from build123d import *

# Parameters (mm, degrees)
F0_R     = 11.176
F1_DEPTH = 19.05
F0_R_2   = 6.35
F2_DEPTH = 12.7
F4_DEPTH = 31.75
F6_DEPTH = 16.002


with BuildPart() as f1:
    # F0 (on Front) → F1 (new body)
    with BuildSketch(Plane.XZ):
        with BuildLine():
            ThreePointArc((-25.4, -44.45), (-17.960512, -62.410512), (0, -69.85))
            ThreePointArc((0, -69.85), (17.960512, -62.410512), (25.4, -44.45))
            Line((25.4, -44.45), (25.4, 44.45))
            ThreePointArc((25.4, 44.45), (17.960512, 62.410512), (0, 69.85))
            ThreePointArc((0, 69.85), (-17.960512, 62.410512), (-25.4, 44.45))
            Line((-25.4, 44.45), (-25.4, -44.45))
        make_face()
        with Locations((0, -44.45)):
            Circle(F0_R, mode=Mode.SUBTRACT)
        with Locations((0, 44.45)):
            Circle(F0_R, mode=Mode.SUBTRACT)
    extrude(amount=F1_DEPTH)

    # F0 (on Front) → F2 (join)
    with BuildSketch(Plane.XZ):
        with Locations((0, -44.45)):
            Circle(F0_R)
        with Locations((0, -44.45)):
            Circle(F0_R_2, mode=Mode.SUBTRACT)
        with Locations((0, 44.45)):
            Circle(F0_R)
        with Locations((0, 44.45)):
            Circle(F0_R_2, mode=Mode.SUBTRACT)
    extrude(amount=F2_DEPTH)

    # F3 (on face) → F4 (join)
    with BuildSketch(Plane.XZ.offset(19.05)):
        with BuildLine():
            ThreePointArc((12.869681, 6.35), (13.975765, 3.260246), (14.351, 0))
            ThreePointArc((14.351, 0), (13.975765, -3.260246), (12.869681, -6.35))
            Line((12.869681, -6.35), (24.593444, -6.35))
            ThreePointArc((24.593444, -6.35), (24.631158, -6.2021), (24.667983, -6.053976))
            ThreePointArc((24.667983, -6.053976), (25.399541, 0.152632), (24.593444, 6.35))
            Line((24.593444, 6.35), (12.869681, 6.35))
        make_face()
        with BuildLine():
            ThreePointArc((6.35, 12.869681), (10.147689, 10.147689), (12.869681, 6.35))
            Line((12.869681, 6.35), (24.593444, 6.35))
            ThreePointArc((24.593444, 6.35), (17.960512, 17.960512), (6.35, 24.593444))
            Line((6.35, 24.593444), (6.35, 12.869681))
        make_face()
        with BuildLine():
            Line((24.593444, -6.35), (12.869681, -6.35))
            ThreePointArc((12.869681, -6.35), (10.147689, -10.147689), (6.35, -12.869681))
            Line((6.35, -12.869681), (6.35, -24.593444))
            ThreePointArc((6.35, -24.593444), (17.960512, -17.960512), (24.593444, -6.35))
        make_face()
        with BuildLine():
            ThreePointArc((-6.35, 12.869681), (0, 14.351), (6.35, 12.869681))
            Line((6.35, 12.869681), (6.35, 24.593444))
            ThreePointArc((6.35, 24.593444), (0, 25.4), (-6.35, 24.593444))
            Line((-6.35, 24.593444), (-6.35, 12.869681))
        make_face()
        with BuildLine():
            Line((6.35, -24.593444), (6.35, -12.869681))
            ThreePointArc((6.35, -12.869681), (0, -14.351), (-6.35, -12.869681))
            Line((-6.35, -12.869681), (-6.35, -24.593444))
            ThreePointArc((-6.35, -24.593444), (0, -25.4), (6.35, -24.593444))
        make_face()
        with BuildLine():
            ThreePointArc((-12.869681, 6.35), (-10.147689, 10.147689), (-6.35, 12.869681))
            Line((-6.35, 12.869681), (-6.35, 24.593444))
            ThreePointArc((-6.35, 24.593444), (-17.943038, 17.977969), (-24.581048, 6.397819))
            ThreePointArc((-24.581048, 6.397819), (-24.587258, 6.373913), (-24.593444, 6.35))
            Line((-24.593444, 6.35), (-12.869681, 6.35))
        make_face()
        with BuildLine():
            Line((-6.35, -24.593444), (-6.35, -12.869681))
            ThreePointArc((-6.35, -12.869681), (-10.147689, -10.147689), (-12.869681, -6.35))
            Line((-12.869681, -6.35), (-24.593444, -6.35))
            ThreePointArc((-24.593444, -6.35), (-17.960512, -17.960512), (-6.35, -24.593444))
        make_face()
        with BuildLine():
            ThreePointArc((-12.869681, -6.35), (-14.351, 0), (-12.869681, 6.35))
            Line((-12.869681, 6.35), (-24.593444, 6.35))
            ThreePointArc((-24.593444, 6.35), (-25.4, 0), (-24.593444, -6.35))
            Line((-24.593444, -6.35), (-12.869681, -6.35))
        make_face()
    extrude(amount=F4_DEPTH)

    # F5 (on face) → F6 (cut)
    with BuildSketch(Plane.XZ.offset(50.8)):
        with BuildLine():
            ThreePointArc((24.667983, -6.053976), (25.399541, 0.152632), (24.593444, 6.35))
            Line((24.593444, 6.35), (12.869681, 6.35))
            ThreePointArc((12.869681, 6.35), (13.975765, 3.260246), (14.351, 0))
            ThreePointArc((14.351, 0), (13.975765, -3.260246), (12.869681, -6.35))
            Line((12.869681, -6.35), (24.593444, -6.35))
            ThreePointArc((24.593444, -6.35), (24.631158, -6.2021), (24.667983, -6.053976))
        make_face()
        with BuildLine():
            ThreePointArc((-12.869681, -6.35), (-14.351, 0), (-12.869681, 6.35))
            Line((-12.869681, 6.35), (-24.593444, 6.35))
            ThreePointArc((-24.593444, 6.35), (-25.4, 0), (-24.593444, -6.35))
            Line((-24.593444, -6.35), (-12.869681, -6.35))
        make_face()
        with BuildLine():
            ThreePointArc((6.35, -12.869681), (0, -14.351), (-6.35, -12.869681))
            Line((-6.35, -12.869681), (-6.35, -24.593444))
            ThreePointArc((-6.35, -24.593444), (0, -25.4), (6.35, -24.593444))
            Line((6.35, -24.593444), (6.35, -12.869681))
        make_face()
        with BuildLine():
            ThreePointArc((6.35, 24.593444), (0, 25.4), (-6.35, 24.593444))
            Line((-6.35, 24.593444), (-6.35, 12.869681))
            ThreePointArc((-6.35, 12.869681), (0, 14.351), (6.35, 12.869681))
            Line((6.35, 12.869681), (6.35, 24.593444))
        make_face()
    extrude(amount=-F6_DEPTH, mode=Mode.SUBTRACT)


solid = f1.part
Here's how the part is built. I have some questions about the finished solid (model axes, mm). A direction names the side the tool comes from. Round coordinates to 2 decimals unless told otherwise and drop trailing zeros. Loops run counter-clockwise (first coordinate to the right, second up) from the corner with the lowest first, then second, coordinate; pieces in that order, holes last. Notation, with made-up numbers: (67, 37) - (79, 37) arc R14 ccw to (79, 64) - close; hole circle Ø3 at (76, 10). An arc over 180 degrees is marked (long way). One line per question, with ' | ' between items. Start each with the question number.
Q1. Will these pins go through, and if not, where does the flat tip stop? pin 1 (6.5 mm diameter, centred on x = -5, z = -45.5, fed in from -Y); pin 2 (3.5 mm diameter, centred on x = 21, y = -43.5, fed in from +Z); pin 3 (9.5 mm diameter, centred on x = -18, y = -40, fed in from +Z); pin 4 (11.5 mm diameter, centred on x = 0, z = 44.45, fed in from +Y).
Q2. I want a section at C-C (y = -46). Write out the boundary of the cut face in (x, z), then the cut area to 3 significant figures.
Q3. We'd pull the mould along Z, two halves only. Please class faces 1 (the flat face through (25.4, -9, -1)), 2 (the cylindrical face through (25.4, -26.8, 0.1)), 3 (the flat face through (5, -12.7, -49)), 4 (the flat face through (19, -43, 6.35)): +Z half, -Z half, draft (parallel to the pull), parting line (faces both ways), or undercut.
Q4. For faces 5 (the flat face through (0, -34.798, -19)), 6 (the flat face through (-19, -43, -6.35)), 7 (the cylindrical face through (-1.45, -15.83, -33.37)), which set-ups out of +Z, -Z, +X, -X, +Y, -Y let a thin tool reach every point of the face, with its end or its side?
Q5. Please list where these lines run through material, in increasing order: line 1 (Z direction, x = -0.5, y = -14.5); line 2 (X direction, y = -4, z = 44); line 3 (X direction, y = -31, z = 0.5). Write a range as [from, to].
Q6. I want a section at B-B (x = -2). Write out the boundary of the cut face in (y, z).
Q7. I want a section at A-A (y = -5.5). Write out the boundary of the cut face in (x, z), then the cut area to 3 significant figures.
Q8. I want a section at D-D (z = 5). Write out the boundary of the cut face in (x, y), then the cut area to 3 significant figures.
Response values:
1) pin 1: stops at y = -12.7 | pin 2: stops at z = 16.57 | pin 3: stops at z = 21.67 | pin 4: passes through
2) outline: (-24.59, -6.35) arc R25.4 ccw to (-6.35, -24.59) - (-6.35, -12.87) arc R14.35 cw to (-12.87, -6.35) - close; (-24.59, 6.35) - (-12.87, 6.35) arc R14.35 cw to (-6.35, 12.87) - (-6.35, 24.59) arc R25.4 ccw to (-24.58, 6.4) arc R24.41 ccw to start; (6.35, -24.59) arc R25.4 ccw to (24.59, -6.35) - (12.87, -6.35) arc R14.35 cw to (6.35, -12.87) - close; (6.35, 12.87) arc R14.35 cw to (12.87, 6.35) - (24.59, 6.35) arc R25.4 ccw to (6.35, 24.59) - close | area: 808 mm²
3) face 1: draft | face 2: parting line | face 3: undercut | face 4: undercut
4) face 5: +Z, -Z, -Y | face 6: +X, -X, -Y | face 7: -Y
5) line 1: z = [-69.85, -55.61], [-33.29, 33.29], [55.61, 69.85] | line 2: x = [-25.4, -6.33], [6.33, 25.4] | line 3: x = [-25.4, -14.34], [14.34, 25.4]
6) outline: (-34.8, -25.32) - (-19.05, -25.32) - (-19.05, -33.45) - (-12.7, -33.45) - (-12.7, -38.42) - (0, -38.42) - (0, 38.42) - (-12.7, 38.42) - (-12.7, 33.45) - (-19.05, 33.45) - (-19.05, 25.32) - (-34.8, 25.32) - (-34.8, 14.21) - (-19.05, 14.21) - (-19.05, -14.21) - (-34.8, -14.21) - close; (-19.05, -69.77) - (0, -69.77) - (0, -50.48) - (-12.7, -50.48) - (-12.7, -55.45) - (-19.05, -55.45) - close; (-19.05, 55.45) - (-12.7, 55.45) - (-12.7, 50.48) - (0, 50.48) - (0, 69.77) - (-19.05, 69.77) - close
7) outline: (-25.4, -44.45) arc R25.4 ccw to (0, -69.85) arc R25.4 ccw to (25.4, -44.45) - (25.4, 44.45) arc R25.4 ccw to (0, 69.85) arc R25.4 ccw to (-25.4, 44.45) - close; hole circle Ø12.7 at (0, -44.45); hole circle Ø12.7 at (0, 44.45) | area: 6,290 mm²
8) outline: (-25.4, -19.05) - (-24.9, -19.05) - (-24.9, -34.8) - (-13.45, -34.8) - (-13.45, -19.05) - (13.45, -19.05) - (13.45, -34.8) - (24.9, -34.8) - (24.9, -19.05) - (25.4, -19.05) - (25.4, 0) - (-25.4, 0) - close | area: 1,330 mm²
